CAD build for the part. Positions are in the model's coordinates, mm. A direction names the side the tool comes from. Coordinates: 2 decimals unless noted, no trailing zeros. Loops run counter-clockwise (first coordinate to the right, second up) from the corner with the lowest first, then second, coordinate; pieces in that order, holes last. Notation, with made-up numbers: M 57,54.5 L 103,54.5 A13 cw 103,77.5 Z; hole C 71,-34 d4. An arc over 180 degrees is marked long. Answer as a JSON object with one key per item and string values. Group by question number.
Autodesk Fusion 360 part; units mm, degrees
sketch "Sketch1" plane through (0, 0, 0) normal (0, 0, 1) x (1, 0, 0)
  circle A0 centre (0, 0) radius 74.6125
  circle A1 centre (0, 62.7602) radius 2.4447
  line L0 (0, 74.6125) -> (0, -74.6125) construction
  line L1 (-74.6125, 0) -> (74.6125, 0) construction
  circle A2 centre (0, -62.7602) radius 2.4447
  circle A3 centre (-62.7602, 0) radius 2.4447
  circle A4 centre (62.7602, 0) radius 2.4447
  circle A5 centre (0, 0) radius 52.867
  dimension "d1" = 149.225
  dimension "d2" = 4.8895
  dimension "d3" = 4.8895
  dimension "d4" = 62.7602
  dimension "d5" = 62.7602
extrude "Extrude1" add sketch "Sketch1" along normal blind 30.48 contours A0 | A1 | A2 | A3 | A4 | A5
extrude "Extrude2" cut sketch "Sketch1" along normal blind 30.48 contours A1 | A2 | A3 | A4
ref_plane "WorkPlane1" through (0, 0, 12.125) normal (-0.7071, 0.7071, 0) x (0, 0, 1)
sketch "Sketch3" plane through (0, 0, 0) normal (-0.7071, 0.7071, 0) x (0, 0, 1)
  circle A0 centre (15.5211, 0) radius 2.4447
  dimension "d12" = 4.8895
  dimension "d29" = 15.5211
extrude "Extrude3" cut sketch "Sketch3" along normal blind 63.5 from surface at 44.1325
extrude "Extrude4" cut sketch "Sketch3" against normal blind 63.5 from surface at -44.1325
ref_plane "WorkPlane2" through (0, 0, 12.125) normal (-0.7071, -0.7071, 0) x (0, 0, 1)
sketch "Sketch4" plane through (0, 0, 0) normal (-0.7071, -0.7071, 0) x (0, 0, 1)
  circle A0 centre (15.551, 0.1414) radius 2.4447
  dimension "d20" = 4.8895
extrude "Extrude5" cut sketch "Sketch4" along normal blind 63.5 from surface at 44.1325
extrude "Extrude6" cut sketch "Sketch4" against normal blind 63.5 from surface at -44.1325
extrude "Extrude7" cut sketch "Sketch1" along normal blind 20.32 contours A5
Item 1: Drill centre lines: L1, parallel to Y at x = 0, z = 7.75; L2, parallel to X at y = 1.5, z = 4.5; L3, parallel to X at y = 40, z = 15.5. Where is each one in solid material? Low to high. Write a range as from..to.
Item 2: Tool access for faces 5 (the flat face through (-1, 1, 20.32)), 6 (the flat face through (16, 51, 0)): list every direction of +Z, -Z, +X, -X, +Y, -Y with a clear straight run to the whole face (end or side of a thin tool).
Item 3: Pull direction Y, two halves, no side cores. Call faces 1 (the flat face through (-1, 1, 30.48)), 2 (the cylindrical face through (-0.53, -60.374, 15.027)), 3 (the cylindrical face through (1.13, 64.93, 15.03)), 4 (the cylindrical face through (-59.21, 45.4, 15.03)): released by +Y, released by -Y, zero draft, split by the parting line, or undercut.
Item 4: Pin check, flat tips, straight feed: pin 1 (5 mm diameter, centred on y = 39, z = 24.5, fed in from -X); pin 2 (4 mm diameter, centred on x = 0, y = -62.76, fed in from +Z); pin 3 (5 mm diameter, centred on x = -52, z = 14.5, fed in from +Y); pin 4 (1.5 mm diameter, centred on x = -30.5, z = 19, fed in from -Y). Stop position of each tip, or through.
Item 5: Slice it at D-D, the plane y = -30.5. Write the cut outline in (x, z), then the cut area to 3 significant figures.
Item 6: Slice it at A-A, the plane y = 0. Write the cut outline in (x, z).
Item 7: Slice it at C-C, the plane z = 8.5. Write the cut outline in (x, y) (1 decimal).
Computed:
{
 "1": {"L1": "-74.61..-65.2, -60.32..-52.87, 52.87..60.32, 65.2..74.61", "L2": "-74.6..-64.69, -60.83..-52.85, 52.85..60.83, 64.69..74.6", "L3": "-62.98..-43.46, -36.54..-34.57, 34.57..36.34, 43.26..62.98"},
 "2": {"face 5": "-Z", "face 6": "-Z, +X, -X, +Y, -Y"},
 "3": {"face 1": "zero draft", "face 2": "undercut", "face 3": "undercut", "face 4": "split by the parting line"},
 "4": {"pin 1": "x = -65.08", "pin 2": "through", "pin 3": "y = 55.83", "pin 4": "y = -68.42"},
 "5": {"outline": "M -68.09,0 L -43.18,0 L -43.18,20.32 L 43.18,20.32 L 43.18,0 L 68.09,0 L 68.09,30.48 L -68.09,30.48 Z", "area": "2,400 mm2"},
 "6": {"outline": "M -74.61,0 L -65.2,0 L -65.2,30.48 L -74.61,30.48 Z; M -60.32,0 L -52.87,0 L -52.87,20.32 L 52.87,20.32 L 52.87,0 L 60.32,0 L 60.32,30.48 L -60.32,30.48 Z; M 65.2,0 L 74.61,0 L 74.61,30.48 L 65.2,30.48 Z"},
 "7": {"outline": "C 0,0 d149.2; hole C -62.8,0 d4.9; hole C 0,0 d105.7; hole C 0,-62.8 d4.9; hole C 0,62.8 d4.9; hole C 62.8,0 d4.9"}
}
